Geometry: final body of the model. Coordinates: model frame, mm. Coordinates: 2 decimals unless noted, no trailing zeros. Loops run counter-clockwise (first coordinate to the right, second up) from the corner with the lowest first, then second, coordinate; pieces in that order, holes last. Notation, with made-up numbers: (-35.75, 71.5) -> (-13.75, 71.5) arc R17 ccw to (-13.75, 98.5) -> close; hole circle Ø10 at (3, 52). An arc over 180 degrees is marked (long way). One line per item, written item: value. Start each with the question number.
from build123d import *


with BuildPart() as part:
    # Sweep2: sweep along a path in Schizzo2
    with BuildLine(Plane(origin=(0, 0, 0), x_dir=(0, 0, -1), z_dir=(1, 0, 0))) as sweep2_path:
        Line((13.145484476, 85.493570144), (267.7362051, 8.553542371))
        ThreePointArc((267.7362051, 8.553542371), (304.754104599, -77.714587953), (213.39832656, -99.316370558))
        Line((213.39832656, -99.316370558), (0.035611501, 59.468246845))
        ThreePointArc((0.035611501, 59.468246845), (-4.343739367, 77.988894569), (13.145484476, 85.493570144))
    # Schizzo3D1 → Sweep2 (sweep)
    with BuildSketch(Plane(origin=(9.500289888, 88.002440666, -22.845650773), x_dir=(-1, 0, 0), z_dir=(0, 0.28929028421703545, 0.9572414175419004))):
        Polygon((0, 0), (19, 0), (17.855289888, 5.20775864), (1.145289888, 5.20775864), align=None)
    sweep(path=sweep2_path.line)


solid = part.part
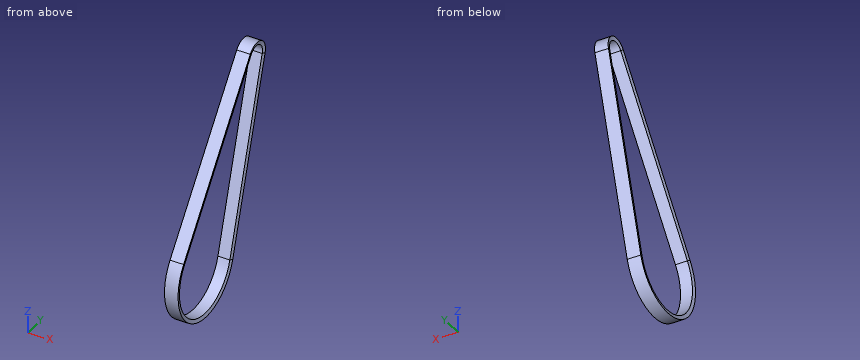
1. Section C-C on y = 32.5. Return the cut outline in (x, z) (3 decimals), plus the area to 3 significant figures.
2. Line query: L1, parallel to Y at x = -4.75, z = -62; L2, parallel to Z at x = -1.5, y = -24; L3, parallel to Y at x = -5, z = -18.5. Output: solid intervals per line, ascending. Write a range as [from, to].
3. Pin query (flat end, axial travel): pin 1 Ø1.5 at (x, z) = (1.5, -281) entering from -Y; pin 2 Ø8 at (y, z) = (7.5, -263) entering from -X; pin 3 Ø3 at (y, z) = (31, -43) entering from -X; pin 4 Ø1 at (x, y) = (-4.5, -20) entering from -Z. Return the tip coordinate at first contact, or that it passes through.
4. Section A-A on z = -63.5. Return the cut outline in (x, y) (3 decimals).
5. Section B-B on x = 4.5. Return the cut outline in (y, z), plus the area to 3 significant figures.
Checks:
1. outline: (-9.5, -206.5) -> (9.5, -206.5) -> (8.355, -188.499) -> (-8.355, -188.499) -> close; (-9.5, -27.551) -> (-8.355, -36.274) -> (8.355, -36.274) -> (9.5, -27.551) -> close
1. area: 477 mm²
2. L1: [6.86, 13.35], [70.73, 76.17]
2. L2: [-311.17, -305.46], [-112.19, -103.47]
2. L3: [39.24, 45.73], [83.88, 89.32]
3. pin 1: y = -109.37
3. pin 2: x = -8.71
3. pin 3: through
3. pin 4: z = -309.55
4. outline: (-9.5, 5.746) -> (9.5, 5.746) -> (8.355, 12.238) -> (-8.355, 12.238) -> close; (-9.5, 75.716) -> (-8.355, 70.276) -> (8.355, 70.276) -> (9.5, 75.716) -> close
5. outline: (-103.49, -210.29) arc R66.52 ccw (long way) to (13.54, -269.24) -> (90.48, -14.65) arc R20 ccw to (55.29, 3.07) -> close; hole (-99.32, -213.4) arc R61.31 ccw (long way) to (8.55, -267.74) -> (85.49, -13.15) arc R14.79 ccw to (59.47, -0.04) -> close
5. area: 4,180 mm²
